Read the model definition and answer for the solid it produces. Units are mm, in the model's axes. A direction names the side the tool comes from. Round coordinates to 2 decimals unless told otherwise and drop trailing zeros. Order: outer loops, then holes, each group sorted by start corner. A loop starts at its lowest first (then second) coordinate and runs counter-clockwise, first axis right, second up. Notation, with made-up numbers: (43, 71) - (60, 71) arc R7 ccw to (60, 80) - close; hole circle Ø6 at (37.25, 24.5). An arc over 180 degrees is marked (long way). Put each result on its own line as item: value. Start each with the question number.
Q1. Section A-A on z = 0 is taken. Give the vertices of the cut face in (x, y).
Q2. For a pull along Y with two mould halves and no side action, classify faces 1 (the face through (0.089, -1.304, -0.383)), 2 (the face through (0, -16, 0)), 3 (the face through (1, -14, 0)) as pulls with the +Y half, pulls with the -Y half, needs draft (parallel to the pull), parting line crosses it, or undercut.
Q3. Section B-B on x = 0 is taken. Give the vertices of the cut face in (y, z), then the cut area to 3 significant figures.
Q4. Find the intervals of material crossed by line 1 along Y through (x, z) = (10.75, -0.75); line 2 along Z through (x, y) = (-1, -3); line 3 along Z through (x, y) = (-4.75, -2.25), in increasing order. Write a range as from..to.
Q5. Section D-D on z = 6.5 is taken. Give the vertices of the cut face in (x, y).
Q6. Which of the six approach directions +Z, -Z, +X, -X, +Y, -Y give full straight-line access (tool end or side, diameter ignored) to faces 4 (the face through (0, -14, 3.75)), 5 (the face through (-6.378, -3, -1)), 6 (the face through (6.378, -3, 1)), 7 (the face through (0.1, -2.5, 7.5))?
Q7. Section C-C on y = -2 is taken. Give the vertices of the cut face in (x, z), then the cut area to 3 significant figures.
Q8. Each of these flat-tipped pins is pushed along its axis until it touches: pin 1 Ø8 at (y, z) = (-13.5, -10) entering from +X; pin 2 Ø3 at (y, z) = (-7, -3) entering from +X; pin 3 Ø4 at (y, z) = (-4, 7) entering from +X. Where does it stop, or does it pass through?
from build123d import *

# Parameters (mm, degrees)
F0_R      = 7.5
F1_DEPTH  = 5
F2_R      = 5
F3_DEPTH  = 7
F4_R      = 12.5
F5_DEPTH  = 1
F6_W      = 2
F6_H      = 7.5
F7_DEPTH  = 3
F9_DEPTH  = 5
F10_R     = 1
F11_DEPTH = 25


with BuildPart() as f1:
    # F0 (on Front) → F1 (new body)
    with BuildSketch(Plane.XZ):
        Circle(F0_R)
    extrude(amount=F1_DEPTH)

    # F2 (on face) → F3 (join)
    with BuildSketch(Plane.XZ.offset(5)):
        Circle(F2_R)
    extrude(amount=F3_DEPTH)

    # F4 (on face) → F5 (join)
    with BuildSketch(Plane.XZ.offset(12)):
        Circle(F4_R)
    extrude(amount=F5_DEPTH)

    # F6 (on face) → F7 (join)
    with BuildSketch(Plane.XZ.offset(13)):
        Rectangle(F6_W, F6_H)
    extrude(amount=F7_DEPTH)

    # F8 (on face) → F9 (cut)
    with BuildSketch(Plane(origin=(0, 0, 0), x_dir=(-1, 0, 0), z_dir=(0, 1, 0))):
        with BuildLine():
            Line((-6.377801, -3.946347), (-6.377801, 3.946347))
            ThreePointArc((-6.377801, 3.946347), (-7.5, 0), (-6.377801, -3.946347))
        make_face()
        with BuildLine():
            ThreePointArc((6.377801, -3.946347), (7.5, 0), (6.377801, 3.946347))
            Line((6.377801, 3.946347), (6.377801, -3.946347))
        make_face()
    extrude(amount=-F9_DEPTH, mode=Mode.SUBTRACT)

    # F10 (on face) → F11 (cut)
    with BuildSketch(Plane.YZ.offset(6.377801)):
        with Locations((-2.22767, 0)):
            Circle(F10_R)
    extrude(amount=-F11_DEPTH, mode=Mode.SUBTRACT)


solid = f1.part
Findings:
1. outline: (-12.5, -13) - (-1, -13) - (-1, -16) - (1, -16) - (1, -13) - (12.5, -13) - (12.5, -12) - (5, -12) - (5, -5) - (6.38, -5) - (6.38, -3.23) - (-6.38, -3.23) - (-6.38, -5) - (-5, -5) - (-5, -12) - (-12.5, -12) - close; (-6.38, -1.23) - (6.38, -1.23) - (6.38, 0) - (-6.38, 0) - close
2. face 1: undercut
2. face 2: pulls with the -Y half
2. face 3: needs draft
3. outline: (-16, -3.75) - (-13, -3.75) - (-13, -12.5) - (-12, -12.5) - (-12, -5) - (-5, -5) - (-5, -7.5) - (0, -7.5) - (0, 7.5) - (-5, 7.5) - (-5, 5) - (-12, 5) - (-12, 12.5) - (-13, 12.5) - (-13, 3.75) - (-16, 3.75) - close; hole circle Ø2 at (-2.23, 0)
3. area: 189 mm2
4. line 1: -13..-12
4. line 2: -7.43..-0.64, 0.64..7.43
4. line 3: -5.8..-1, 1..5.8
5. outline: (-10.68, -13) - (10.68, -13) - (10.68, -12) - (-10.68, -12) - close; (-3.74, -5) - (3.74, -5) - (3.74, 0) - (-3.74, 0) - close
6. face 4: +Z, +X, -X, -Y
6. face 5: +Z, -Z, -X, +Y
6. face 6: +Z, -Z, +X, +Y
6. face 7: +Z, +Y
7. outline: (-6.38, -3.95) arc R7.5 ccw to (6.38, -3.95) - (6.38, -0.97) - (-6.38, -0.97) - close; (-6.38, 0.97) - (6.38, 0.97) - (6.38, 3.95) arc R7.5 ccw to (-6.38, 3.95) - close
7. area: 140 mm2
8. pin 1: x = 10.95
8. pin 2: x = 4.77
8. pin 3: x = 5.59
